from build123d import *

# Parameters (mm, degrees)
SKETCH2_W          = 22
SKETCH2_H          = 56
CUT_EXTRUDE1_DEPTH = 16
SKETCH3_W          = 22
SKETCH3_H          = 43
CUT_EXTRUDE2_DEPTH = 36
SKETCH5_R          = 12.5
CUT_EXTRUDE4_DEPTH = 16
SKETCH6_W          = 22
SKETCH6_H          = 30
CUT_EXTRUDE5_DEPTH = 97.474089786
SKETCH4_R          = 2.13
CUT_EXTRUDE3_DEPTH = 10


with BuildPart() as part:
    # Sketch1 → Revolve1 (revolve)
    with BuildSketch(Plane.XY, mode=Mode.PRIVATE) as revolve1_sk:
        Polygon((0, 0), (45, 0), (50, 5), (50, 50), (45, 55), (0, 55), align=None)
    revolve(revolve1_sk.sketch.rotate(Axis((0, 55, 0), (0, -1, 0)), 180), axis=Axis((0, 55, 0), (0, -1, 0)))

    # Sketch2 → Cut-Extrude1 (cut)
    with BuildSketch(Plane.XZ):
        with Locations((0, -10)):
            Rectangle(SKETCH2_W, SKETCH2_H)
    extrude(amount=-CUT_EXTRUDE1_DEPTH, mode=Mode.SUBTRACT)

    # Sketch3 → Cut-Extrude2 (cut)
    with BuildSketch(Plane.XZ.offset(-16)):
        with Locations((0, -10)):
            Rectangle(SKETCH3_W, SKETCH3_H)
    extrude(amount=-CUT_EXTRUDE2_DEPTH, mode=Mode.SUBTRACT)

    # Sketch5 → Cut-Extrude4 (cut)
    with BuildSketch(Plane(origin=(0, 0, 0), x_dir=(1, 0, 0), z_dir=(0, 1, 0))):
        Circle(SKETCH5_R)
    extrude(amount=CUT_EXTRUDE4_DEPTH, mode=Mode.SUBTRACT)

    # Sketch6 → Cut-Extrude5 (cut, through all)
    with BuildSketch(Plane(origin=(0, 0, 11.5), x_dir=(-1, 0, 0), z_dir=(0, 0, -1))):
        with Locations((0, 37)):
            Rectangle(SKETCH6_W, SKETCH6_H)
    extrude(amount=-CUT_EXTRUDE5_DEPTH, mode=Mode.SUBTRACT)

    # Sketch4 → Cut-Extrude3 (cut)
    with BuildSketch(Plane.XZ.offset(-16)):
        with Locations((-5, 14.65)):
            Circle(SKETCH4_R)
        with Locations(Location((5, 14.65, 0), (0, 0, 270))):
            Circle(SKETCH4_R)
        with Locations((5, -34.85)):
            Circle(SKETCH4_R)
        with Locations(Location((-5, -34.85, 0), (0, 0, 180))):
            Circle(SKETCH4_R)
    extrude(amount=-CUT_EXTRUDE3_DEPTH, mode=Mode.SUBTRACT)


solid = part.part
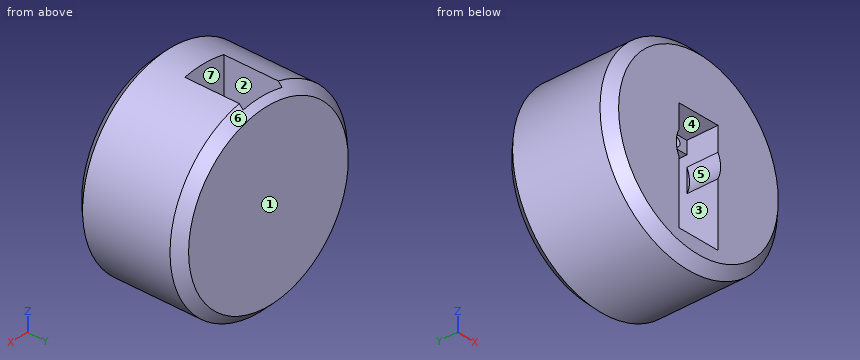
Input: part model. Units: mm. Frame: model coordinates. Face numbers are marked on the shaded views. A direction names the side the tool comes from. Give positions to 0.01 mm unless a question says otherwise; leave off trailing zeros. Write each loop counter-clockwise with the first axis right and the second up, starting at its lowest first coordinate (ties: lowest second). Pieces come first, ordered by that corner, then holes.
Q1. Section B-B, the plane z = 0. Output: boundary loops of the cut face in (x, y), plus the area to 3 significant figures.
Q2. Section D-D, the plane y = 39. Output: boundary loops of the cut face in (x, z) (3 decimals).
Q3. Section C-C, the plane y = 24. Output: boundary loops of the cut face in (x, z) (3 decimals).
Q4. Set-up query: the marked faces 5, 6 and 7. Return all of +Z, -Z, +X, -X, +Y, -Y with unobstructed straight access to the full face (end or side cutting, diameter ignored); none if empty.
Q5. Section A-A, the plane x = 0. Output: boundary loops of the cut face in (y, z).
Q6. Material intervals for probe 1 along Z at (x, y) = (-5, 21); probe 2 along X at (y, z) = (18, -34); probe 3 along X at (y, z) = (20, 14), sorted ascending.
Q7. Pull-direction query (Y, two-part tool) for the marked faces 1, 2, 3 and 4; classes: pulls with the +Y half, pulls with the -Y half, needs draft (parallel to the pull), parting line crosses it, or undercut.
Q8. First-contact query: P1, Ø5, axis at x = 5, z = 16, coming from the -Y side; P2, Ø1.5, axis at y = 9.5, z = 4.5, coming from the -X side; P3, Ø3, axis at x = -24, y = 10, coming from the -Z side; P4, Ø8, axis at y = 19.5, z = -9.5, coming from the +X side. Flat tips, straight axial feed; report the tip coordinate or a pass-through.
Filled in:
1. outline: (-50, 5) - (-45, 0) - (-12.5, 0) - (-12.5, 16) - (-11, 16) - (-11, 52) - (11, 52) - (11, 16) - (12.5, 16) - (12.5, 0) - (45, 0) - (50, 5) - (50, 50) - (45, 55) - (-45, 55) - (-50, 50) - close
1. area: 4,260 mm2
2. outline: (-11, -31.5) - (-11, 48.775) arc R50 ccw (long way) to (11, 48.775) - (11, -31.5) - close
3. outline: (-11, -31.5) - (-11, 48.775) arc R50 ccw (long way) to (11, 48.775) - (11, -31.5) - close; hole circle Ø4.26 at (-5, -34.85); hole circle Ø4.26 at (5, -34.85)
4. face 5: -Y
4. face 6: +Y
4. face 7: +Z
5. outline: (0, -45) - (5, -50) - (50, -50) - (55, -45) - (55, 45) - (52, 48) - (52, -31.5) - (16, -31.5) - (16, -38) - (0, -38) - close; (0, 18) - (16, 18) - (16, 11.5) - (22, 11.5) - (22, 50) - (5, 50) - (0, 45) - close
6. probe 1: z = -49.75 to -36.98, -32.72 to -31.5, 11.5 to 12.52, 16.78 to 49.75
6. probe 2: x = -36.66 to -6.95, -3.05 to 3.05, 6.95 to 36.66
6. probe 3: x = -48 to -7.03, -2.97 to 2.97, 7.03 to 48
7. face 1: pulls with the +Y half
7. face 2: undercut
7. face 3: undercut
7. face 4: needs draft
8. P1: stops at y = 0
8. P2: stops at x = -49.86
8. P3: stops at z = -44.65
8. P4: stops at x = 49.7
